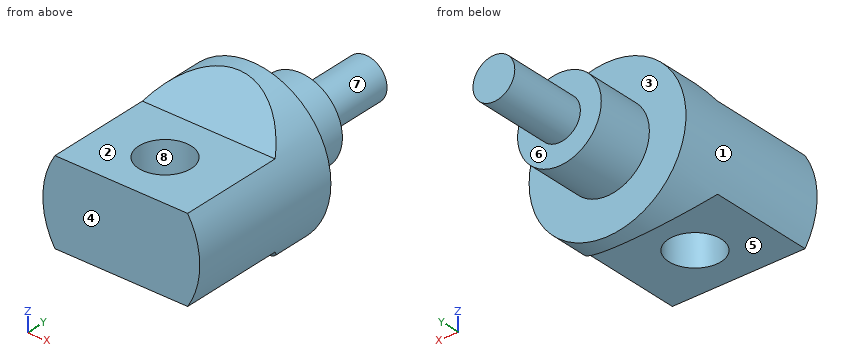
from build123d import *

# Parameters (mm, degrees)
F0_R      = 15
F1_DEPTH  = 30
F3_W      = 30
F3_H      = 20
F4_DEPTH  = 7
F6_W      = 30
F6_H      = 20
F7_DEPTH  = 7
F10_DEPTH = 30
F11_R     = 8
F12_DEPTH = 11
F13_R     = 4
F14_DEPTH = 15
F15_R     = 5
F16_DEPTH = 23.001


with BuildPart() as f1:
    # F0 (on Front) → F1 (new body)
    with BuildSketch(Plane.XZ):
        Circle(F0_R)
    extrude(amount=F1_DEPTH)

    # F3 (on offset) → F4 (cut)
    with BuildSketch(Plane.XY.offset(15)):
        with Locations((0, -20)):
            Rectangle(F3_W, F3_H)
    extrude(amount=-F4_DEPTH, mode=Mode.SUBTRACT)

    # F6 (on offset) → F7 (cut)
    with BuildSketch(Plane.XY.offset(-15)):
        with Locations((0, -20)):
            Rectangle(F6_W, F6_H)
    extrude(amount=F7_DEPTH, mode=Mode.SUBTRACT)

    # F9 (on offset) → F10 (cut)
    with BuildSketch(Plane.YZ.offset(15)):
        Polygon((-3, 15), (-10, 15), (-10, 8), align=None)
        Polygon((-10, -15), (-3, -15), (-10, -8), align=None)
    extrude(amount=-F10_DEPTH, mode=Mode.SUBTRACT)

    # F11 (on face) → F12 (join)
    with BuildSketch(Plane(origin=(0, 0, 0), x_dir=(-1, 0, 0), z_dir=(0, 1, 0))):
        Circle(F11_R)
    extrude(amount=F12_DEPTH)

    # F13 (on face) → F14 (join)
    with BuildSketch(Plane(origin=(0, 11, 0), x_dir=(-1, 0, 0), z_dir=(0, 1, 0))):
        Circle(F13_R)
    extrude(amount=F14_DEPTH)

    # F15 (on face) → F16 (cut, through all)
    with BuildSketch(Plane.XY.offset(8)):
        with Locations((0, -20)):
            Circle(F15_R)
    extrude(amount=-F16_DEPTH, mode=Mode.SUBTRACT)


solid = f1.part
Input: part model. Units: mm. Frame: model coordinates. Face numbers are marked on the shaded views. A direction names the side the tool comes from. Coordinates: 2 decimals unless noted, no trailing zeros. Order: outer loops, then holes, each group sorted by start corner. A loop starts at its lowest first (then second) coordinate and runs counter-clockwise, first axis right, second up. Notation, with made-up numbers: M 45.25,31.5 L 92.25,31.5 A17 ccw 92.25,37.5 Z; hole C 76.25,70.25 d2. An arc over 180 degrees is marked long. Answer in a Markdown table with one row per item.
(1) Section query C-C, the plane y = -20. Output: boundary loops of the cut face in (x, z), plus the area to 3 significant figures.
Numbers:
| item | result |
|---|---|
| outline | M -12.69,-8 L -5,-8 L -5,8 L -12.69,8 A15 ccw Z; M 5,-8 L 12.69,-8 A15 ccw 12.69,8 L 5,8 Z |
| area | 296 mm^2 |
(2) Draft query along Y for the marked faces 6, 7 and 8. Return one class per face: pulls with the +Y half, pulls with the -Y half, needs draft (parallel to the pull), parting line crosses it, or undercut.
Numbers:
| item | result |
|---|---|
| face 6 | pulls with the +Y half |
| face 7 | needs draft |
| face 8 | undercut |
(3) Contact query for flat-ended pins moving along their axis: pin 1 Ø8 at (y, z) = (-7, -7.5) entering from +X; pin 2 Ø8 at (x, y) = (5.5, -16) entering from -Z; pin 3 Ø11.5 at (x, y) = (0, -20) entering from +Z. Output: stop coordinate, or through.
Numbers:
| item | result |
|---|---|
| pin 1 | stops at x = 14.59 |
| pin 2 | stops at z = -8 |
| pin 3 | stops at z = 8 |
(4) Section query A-A, the plane x = 0. Output: boundary loops of the cut face in (y, z).
Numbers:
| item | result |
|---|---|
| outline | M -30,-8 L -25,-8 L -25,8 L -30,8 Z; M -15,-8 L -10,-8 L -3,-15 L 0,-15 L 0,-8 L 11,-8 L 11,-4 L 26,-4 L 26,4 L 11,4 L 11,8 L 0,8 L 0,15 L -3,15 L -10,8 L -15,8 Z |
(5) Material intervals for line 1 (Y direction, x = 0, z = -3.5); line 2 (Z direction, x = -10.75, y = -14); line 3 (X direction, y = -23.5, z = -3), sorted ascending. Write a range as [from, to].
Numbers:
| item | result |
|---|---|
| line 1 | y = [-30, -25], [-15, 26] |
| line 2 | z = [-8, 8] |
| line 3 | x = [-14.7, -3.57], [3.57, 14.7] |
(6) Section query B-B, the plane z = 0. Output: boundary loops of the cut face in (x, y), plus the area to 3 significant figures.
Numbers:
| item | result |
|---|---|
| outline | M -15,-30 L 15,-30 L 15,0 L 8,0 L 8,11 L 4,11 L 4,26 L -4,26 L -4,11 L -8,11 L -8,0 L -15,0 Z; hole C 0,-20 d10 |
| area | 1,120 mm^2 |
(7) Access query for the marked faces 1, 2, 3, 4 and 5. Directions: +Z, -Z, +X, -X, +Y, -Y. A direction counts if a zero-diameter tool reaches every point of the face in a straight line with its end or side. Return the directions, or none.
Numbers:
| item | result |
|---|---|
| face 1 | +Y, -Y |
| face 2 | +Z, +X, -X, -Y |
| face 3 | +Y |
| face 4 | +Z, -Z, +X, -X, -Y |
| face 5 | -Z, +X, -X, -Y |
(8) Section query D-D, the plane x = -10.25. Output: boundary loops of the cut face in (y, z).
Numbers:
| item | result |
|---|---|
| outline | M -30,-8 L -10,-8 L -7.05,-10.95 L 0,-10.95 L 0,10.95 L -7.05,10.95 L -10,8 L -30,8 Z |
